CAD build for the part. Positions are in the model's coordinates, mm. Face numbers are marked on the shaded views. A direction names the side the tool comes from. Give positions to 0.01 mm unless a question says otherwise; leave off trailing zeros. Write each loop counter-clockwise with the first axis right and the second up, starting at its lowest first coordinate (ties: lowest second). Pieces come first, ordered by that corner, then holes. Notation, with made-up numbers: (-3.75, 88.25) - (43.25, 88.25) arc R37 cw to (43.25, 125.25) - close; hole circle Ø10 at (21, 82). An arc over 180 degrees is marked (long way). Answer as a JSON object with one key per item and string values.
from build123d import *

# Parameters (mm, degrees)
SKETCH1_R           = 2.75
BOSS_EXTRUDE1_DEPTH = 30
SKETCH4_W           = 7
SKETCH4_H           = 20
SKETCH4_W_2         = 13.969977059
CUT_EXTRUDE2_DEPTH  = 34


with BuildPart() as part:
    # Sketch1 → Boss-Extrude1 (new body)
    with BuildSketch(Plane(origin=(0, 0, 0), x_dir=(1, 0, 0), z_dir=(0, 1, 0))):
        with BuildLine():
            Line((-46.676005757, -6.723173527), (3.323994243, 17.99725225))
            ThreePointArc((3.323994243, 17.99725225), (6.37102648, 20.763151262), (7.5, 24.720425777))
            Line((7.5, 24.720425777), (7.5, 114.720425777))
            ThreePointArc((7.5, 114.720425777), (1.53049147, 122.062605008), (-6.875358896, 117.716997159))
            Line((-6.875358896, 117.716997159), (-56.875358896, 2.996571382))
            ThreePointArc((-56.875358896, 2.996571382), (-55.174109392, -5.429419122), (-46.676005757, -6.723173527))
        make_face()
        with Locations((-50, 0)):
            Circle(SKETCH1_R, mode=Mode.SUBTRACT)
        Polygon((-7.5, 29.378946496), (-45.351897452, 10.664646067), (-15.254476159, 79.720425777), (-7.5, 79.720425777), align=None, mode=Mode.SUBTRACT)
        with Locations((0, 54.720425777)):
            Circle(SKETCH1_R, mode=Mode.SUBTRACT)
        with Locations((-17.304325397, 84.720425777)):
            Circle(SKETCH1_R, mode=Mode.SUBTRACT)
        with Locations((0, 84.720425777)):
            Circle(SKETCH1_R, mode=Mode.SUBTRACT)
        Polygon((-10.8960544, 89.720425777), (0, 114.720425777), (0, 89.720425777), align=None, mode=Mode.SUBTRACT)
        with Locations((0, 24.720425777)):
            Circle(SKETCH1_R, mode=Mode.SUBTRACT)
    extrude(amount=BOSS_EXTRUDE1_DEPTH)

    # Sketch4 → Cut-Extrude2 (cut)
    with BuildSketch(Plane(origin=(-48.89363441, 0, -21.309908013), x_dir=(-0.399542851, 0, 0.91671452), z_dir=(-0.91671452, 0, -0.399542851))):
        with Locations((16.477142547, 15)):
            Rectangle(SKETCH4_W, SKETCH4_H)
        with Locations((26.962131077, 15)):
            Rectangle(SKETCH4_W_2, SKETCH4_H)
    extrude(amount=-CUT_EXTRUDE2_DEPTH, mode=Mode.SUBTRACT)


solid = part.part
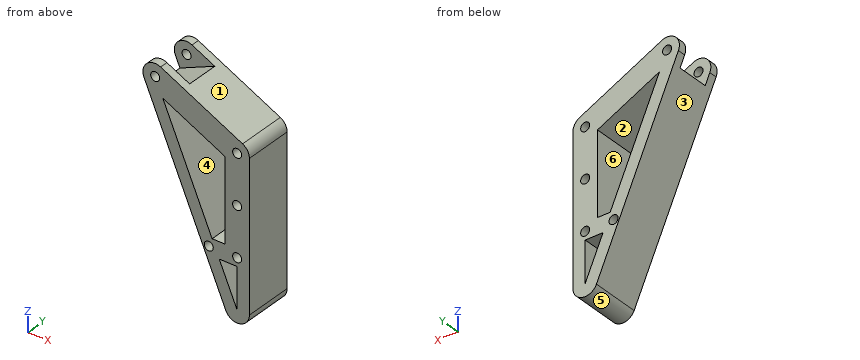
(1) Saw through at C-C, the plane y = 7.75. Give the cut face in (x, z), and give its area (3 significant figures).
Answer key:
{"outline": "(-54.08, -9.41) - (-6.88, -117.72) arc R7.5 ccw to (7.5, -114.72) - (7.5, -24.72) arc R7.5 ccw to (3.32, -18) - (-32.8, -0.14) - close; hole (-45.35, -10.66) - (-15.25, -79.72) - (-7.5, -79.72) - (-7.5, -29.38) - close; hole circle Ø5.5 at (-17.3, -84.72); hole (-10.9, -89.72) - (0, -114.72) - (0, -89.72) - close; hole circle Ø5.5 at (0, -84.72); hole circle Ø5.5 at (0, -54.72); hole circle Ø5.5 at (0, -24.72)", "area": "2,770 mm²"}
(2) Pull direction X, two halves, no side cores. Call the marked faces 1, 2, 3 and 4: pulls with the +X half, pulls with the -X half, needs draft (parallel to the pull), parting line crosses it, or undercut.
Answer key:
{"face 1": "pulls with the +X half", "face 2": "undercut", "face 3": "pulls with the -X half", "face 4": "undercut"}
(3) Saw through at B-B, the plane z = -65. Give the cut face in (x, y).
Answer key:
{"outline": "(-29.85, 0) - (-21.67, 0) - (-21.67, 30) - (-29.85, 30) - close; (-7.5, 0) - (7.5, 0) - (7.5, 30) - (-7.5, 30) - close"}
(4) Probe L1, parallel to X at y = 7.75, z = -79; L2, parallel to Z at x = -31, y = 24.5; L3, parallel to Z at x = -24, y = 5. List the from-to ranges inside material, lowest first. Write a range as [from, to].
Answer key:
{"L1": "x = [-23.75, -15.57], [-7.5, 7.5]", "L2": "z = [-62.37, -43.59], [-17.76, -1.03]", "L3": "z = [-78.43, -59.65], [-21.22, -4.49]"}
(5) Flat gauge pins, fed straight in: P1, Ø6, axis at x = -23.5, y = 21.5, coming from the -Z side; P2, Ø5, axis at x = -17.5, z = -96.5, coming from the -Y side; P3, Ø6, axis at y = 22.5, z = -58.5, coming from the -X side; P4, Ø6, axis at x = -10, y = 8, coming from the +Z side. Where does each tip first touch, or does it go through?
Answer key:
{"P1": "stops at z = -86.46", "P2": "stops at y = 0", "P3": "stops at x = -33.99", "P4": "stops at z = -9.93"}
(6) Saw through at A-A, the plane x = -34.5. Give the cut face in (y, z), and give its area (3 significant figures).
Answer key:
{"outline": "(0, -54.33) - (30, -54.33) - (30, -35.56) - (0, -35.56) - close; (0, -16.03) - (30, -16.03) - (30, 0.7) - (25, 0.7) - (25, -0.88) - (5, -0.88) - (5, 0.7) - (0, 0.7) - close", "area": "1,030 mm²"}
(7) Saw through at D-D, the plane x = -50. Give the cut face in (y, z), and give its area (3 significant figures).
Answer key:
{"outline": "(0, -18.77) - (30, -18.77) - (30, -2.75) - (25, -2.75) - (25, -7.64) - (5, -7.64) - (5, -2.75) - (0, -2.75) - close; (0, 2.75) - (5, 2.75) - (5, 7.5) - (0, 7.5) - close; (25, 2.75) - (30, 2.75) - (30, 7.5) - (25, 7.5) - close", "area": "430 mm²"}
(8) 3-axis set-ups, long thin cutter, end or side, ignore diameter. For the marked faces 5 and 6: which of +Z, -Z, +X, -X, +Y, -Y reach the whole face in a straight line?
Answer key:
{"face 5": "-Z, +Y, -Y", "face 6": "+Y, -Y"}
